For this review, take the finished solid that the model builds, in its own axes (mm). A direction names the side the tool comes from. Give positions to 0.01 mm unless a question says otherwise; leave off trailing zeros. Loops run counter-clockwise (first coordinate to the right, second up) from the corner with the lowest first, then second, coordinate; pieces in that order, holes last. Notation, with made-up numbers: (11.5, 56.5) - (45.5, 56.5) arc R5 ccw to (45.5, 63.5) - close; hole circle Ø3 at (3.25, 37.25). An arc over 180 degrees is marked (long way). Answer as CSV lines item,"result".
from build123d import *

# Parameters (mm, degrees)
ESBO_O1_R                            = 14.5
RESSALTO_EXTRUS_O1_DEPTH             = 26
ESBO_O2_R                            = 10.5
CORTE_EXTRUS_O2_DEPTH                = 13
FURO_ROSCADO_DE_M22X1_51_D           = 20.5
FURO_ROSCADO_DE_M22X1_51_CSINK_D     = 22.05
FURO_ROSCADO_DE_M22X1_51_CSINK_ANGLE = 90


# Read off the part's stored shape, not the designer's step: Furo roscado de M51
with BuildPart() as part:
    # Esboço1 → Ressalto-extrusão1 (new body)
    with BuildSketch(Plane(origin=(0, 0, 0), x_dir=(1, 0, 0), z_dir=(0, 1, 0))):
        with Locations(Location((0, 0, 0), (0, 0, 90))):
            Circle(ESBO_O1_R)
    extrude(amount=RESSALTO_EXTRUS_O1_DEPTH)

    # Esboço2 → Corte-extrusão2 (cut)
    with BuildSketch(Plane.XZ):
        with Locations(Location((0, 0, 0), (0, 0, 270))):
            Circle(ESBO_O2_R)
    extrude(amount=-CORTE_EXTRUS_O2_DEPTH, mode=Mode.SUBTRACT)

    # Furo roscado de M22x1.51 (through all)
    with Locations(Plane(origin=(0, 26, 0), x_dir=(1, 0, 0), z_dir=(0, 1, 0))):
        with Locations((0, 0)):
            CounterSinkHole(FURO_ROSCADO_DE_M22X1_51_D / 2, FURO_ROSCADO_DE_M22X1_51_CSINK_D / 2, counter_sink_angle=FURO_ROSCADO_DE_M22X1_51_CSINK_ANGLE)

    # Furo roscado de M51 outline → Furo roscado de M51 (revolve, cut)
    with BuildSketch(Plane(origin=(0, 5.075943164, 0), x_dir=(0, 1, 0), z_dir=(0.000288160587710413, 0, -0.999999958481737))):
        Polygon((2.525059426, 14.500059426), (0, 14.500059426), (0, 10.287739691), (2.1, 10.287739691), (2.1, 14.075), align=None)
    revolve(axis=Axis((0, 5.075943164, 0), (0.999999958481737, 0, 0.000288160587710413)), mode=Mode.SUBTRACT)


solid = part.part
1) Consider section C-C on z = -11.5. Write out the cut boundary in (x, y).
From the geometry:
outline,"(-8.83, 0) - (8.83, 0) - (8.83, 26) - (-8.83, 26) - close"
2) Wall thickness on line 1 (X direction, y = 8.5, z = 0); line 2 (X direction, y = 21, z = -4.5); line 3 (Z direction, x = 2.25, y = 21): over which ranges is each line inside the solid? List them lowest first. Write a range as from..to.
From the geometry:
line 1,"x = -14.5..-10.5, 10.5..14.5"
line 2,"x = -13.78..-9.21, 9.21..13.78"
line 3,"z = -14.32..-10, 10..14.32"
3) Machinability: for faces 1 (the flat face through (-11, 26, 2)), 2 (the cylindrical face through (-10.25, 6.41, 2.28)), which of the approach directions +Z, -Z, +X, -X, +Y, -Y give a long, thin tool a straight path to every point of the face, cutting with its end or side? Answer none if there is none.
From the geometry:
face 1,"+Z, -Z, +X, -X, +Y"
face 2,"-Y"
4) Draft analysis for pull direction X (two halves, no side actions). For faces 3 (the cylindrical face through (5.554, 12.818, -13.394)), 4 (the cylindrical face through (12.21, 7.08, 0.63)), 5 (the flat face through (-4, 0, -10)), 6 (the cylindrical face through (2.222, 19.027, 10.006)), state which applies: pulls with the +X half, pulls with the -X half, needs draft (parallel to the pull), parting line crosses it, or undercut.
From the geometry:
face 3,"parting line crosses it"
face 4,"undercut"
face 5,"needs draft"
face 6,"undercut"
5) Consider section B-B on y = 24.25. Write out the cut boundary in (x, z).
From the geometry:
outline,"circle Ø29 at (0, 0); hole circle Ø20.5 at (0, 0)"
6) Consider section D-D on y = 9.75. Write out the cut boundary in (x, z), and give its area (3 significant figures).
From the geometry:
outline,"circle Ø29 at (0, 0); hole circle Ø21 at (0, 0)"
area,"314 mm^2"
7) Consider section A-A on x = 0. Write out the cut boundary in (y, z) (3 decimals), and give its area (3 significant figures).
From the geometry:
outline,"(0, -14.5) - (26, -14.5) - (26, -11.025) - (25.225, -10.25) - (13, -10.25) - (13, -10.5) - (0, -10.5) - close; (0, 10.5) - (13, 10.5) - (13, 10.25) - (25.225, 10.25) - (26, 11.025) - (26, 14.5) - (0, 14.5) - close"
area,"214 mm^2"
8) Insertion check: P1, Ø12.5, axis at x = 0, z = 0, coming from the +Y side; P2, Ø5, axis at y = 4, z = 5, coming from the +X side; P3, Ø4, axis at y = 15, z = 7, coming from the +X side; P4, Ø6, axis at y = 16.5, z = -8, coming from the -X side. Each pin has a flat end and moves straight along its axis. Give the tip position at first contact, or say it passes through.
From the geometry:
P1,"passes through"
P2,"stops at x = 14.28"
P3,"stops at x = 13.61"
P4,"stops at x = -13.61"
